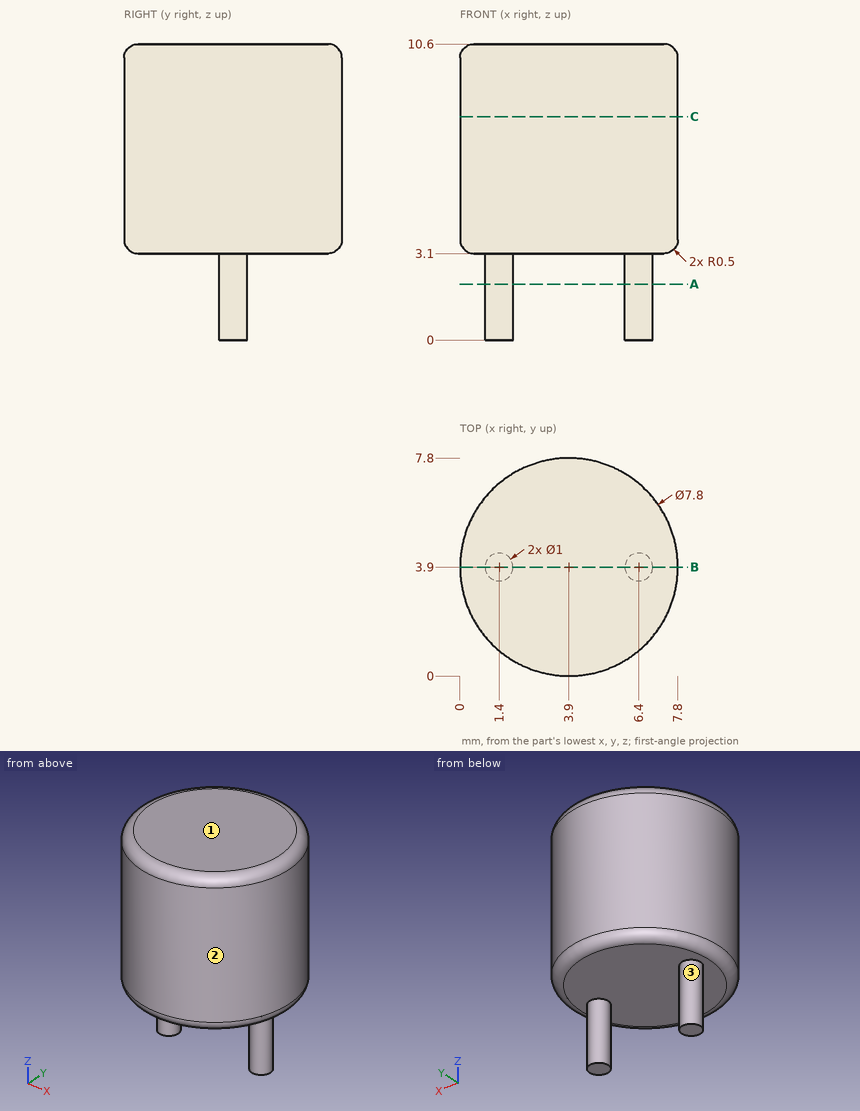
Study the drawing (mm; zero at the part's minimum x, y, z) and answer. Round coordinates to 2 decimals unless told otherwise and drop trailing zeros. Order: outer loops, then holes, each group sorted by start corner. A loop starts at its lowest first (then second) coordinate and runs counter-clockwise, first axis right, second up. Notation, with made-up numbers: (-6, -26.75) -> (42, -26.75) arc R28 cw to (42, 6.25) -> close; hole circle Ø1 at (27.5, 36.5). An arc over 180 degrees is marked (long way). Write each question's results on one line, items separated by ' | '. Start each with the question number.
Q1. Find section B-B (y = 3.9). Determine the outline of the cut face in (x, z).
Q2. Find section C-C (z = 8). Determine the outline of the cut face in (x, y), then the cut area to 3 significant figures.
Q3. Straight lines are drawn through the part: probe 1 along Z at (x, y) = (3.75, 0.5); probe 2 along X at (y, z) = (7.25, 8); probe 3 along X at (y, z) = (3.75, 2). For each, find the intervals that lie inside material, in ascending order. Write a range as from..to.
Q4. Find section A-A (z = 2). Determine the outline of the cut face in (x, y).
Q5. The mould has two halves that part along X. Classify the marked faces 1, 2 and 3: pulls with the +X half, pulls with the -X half, needs draft (parallel to the pull), parting line crosses it, or undercut.
Q6. Each of these flat-tipped pins is pushed along its axis until it touches: pin 1 (4 mm diameter, centred on x = 2, y = 1, fed in from -Z); pin 2 (2 mm diameter, centred on y = 6.5, z = 9, fed in from +X); pin 3 (1 mm diameter, centred on x = 6.5, z = 6, fed in from +Y). Where does it stop, or does it pass through?
Worked answers:
1) outline: (0, 3.6) arc R0.5 ccw to (0.5, 3.1) -> (0.9, 3.1) -> (0.9, 0) -> (1.9, 0) -> (1.9, 3.1) -> (5.9, 3.1) -> (5.9, 0) -> (6.9, 0) -> (6.9, 3.1) -> (7.3, 3.1) arc R0.5 ccw to (7.8, 3.6) -> (7.8, 10.1) arc R0.5 ccw to (7.3, 10.6) -> (0.5, 10.6) arc R0.5 ccw to (0, 10.1) -> close
2) outline: circle Ø7.8 at (3.9, 3.9) | area: 47.8 mm2
3) probe 1: z = 3.1..10.6 | probe 2: x = 1.9..5.9 | probe 3: x = 0.92..1.88, 5.92..6.88
4) outline: circle Ø1 at (1.4, 3.9); circle Ø1 at (6.4, 3.9)
5) face 1: needs draft | face 2: parting line crosses it | face 3: undercut
6) pin 1: stops at z = 3.1 | pin 2: stops at x = 7.46 | pin 3: stops at y = 7.19
